Geometry: final body of the model. Coordinates: model frame, mm. A direction names the side the tool comes from. Coordinates: 2 decimals unless noted, no trailing zeros. Write each loop counter-clockwise with the first axis right and the second up, starting at its lowest first coordinate (ties: lowest second). Pieces come first, ordered by that corner, then holes. Notation, with made-up numbers: (75.5, 81.5) -> (124.5, 81.5) arc R20 ccw to (124.5, 88.5) -> close; hole circle Ø4 at (49.25, -35). An arc over 180 degrees is marked (long way). One line per item, written item: value.
```python
from build123d import *

# Parameters (mm, degrees)
EXTRUDE_1_DEPTH                = 15
SKETCH_2_R                     = 1.5
EXTRUDE_2_DEPTH                = 6
SKETCH_3_R                     = 1.5
SKETCH_3_R_2                   = 1.25
CUT_EXTRUDE_3_DEPTH            = 0.5
CHAMFER_1_SIZE                 = 0.2
M4_CLEARANCE_HOLE1_D           = 2.5
M4_CLEARANCE_HOLE1_DEPTH       = 6
M4_CLEARANCE_HOLE1_CSINK_D     = 3
M4_CLEARANCE_HOLE1_CSINK_ANGLE = 90
M4_CLEARANCE_HOLE1_TIP         = 0.751075774


with BuildPart() as part:
    # Эскиз1 → Вытянуть1 (new body)
    with BuildSketch(Plane.XY):
        Polygon((0, 2.886751346), (-2.5, 1.443375673), (-2.5, -1.443375673), (0, -2.886751346), (2.5, -1.443375673), (2.5, 1.443375673), align=None)
    extrude(amount=EXTRUDE_1_DEPTH)

    # Эскиз2 → Вытянуть2 (add)
    with BuildSketch(Plane.XY.offset(15)):
        Circle(SKETCH_2_R)
    extrude(amount=EXTRUDE_2_DEPTH)

    # Эскиз3 → Вырез-Вытянуть3 (cut)
    with BuildSketch(Plane.XY.offset(15)):
        Circle(SKETCH_3_R)
        Circle(SKETCH_3_R_2, mode=Mode.SUBTRACT)
    extrude(amount=CUT_EXTRUDE_3_DEPTH, mode=Mode.SUBTRACT)

    # Фаска1
    chamfer_1_edges = [part.edges().sort_by_distance(p)[0] for p in [
        (-1.5, 0, 21),
        (-1.5, 0, 15.5),
    ]]
    chamfer(chamfer_1_edges, length=CHAMFER_1_SIZE)

    # M4 Clearance Hole1
    with Locations(Plane(origin=(0, 0, 0), x_dir=(-1, 0, 0), z_dir=(0, 0, -1))):
        with Locations((0, 0)):
            CounterSinkHole(M4_CLEARANCE_HOLE1_D / 2, M4_CLEARANCE_HOLE1_CSINK_D / 2, depth=M4_CLEARANCE_HOLE1_DEPTH, counter_sink_angle=M4_CLEARANCE_HOLE1_CSINK_ANGLE)
            with Locations((0, 0, -(M4_CLEARANCE_HOLE1_DEPTH + M4_CLEARANCE_HOLE1_TIP / 2))):  # 118° drill point
                Cone(0, M4_CLEARANCE_HOLE1_D / 2, M4_CLEARANCE_HOLE1_TIP, mode=Mode.SUBTRACT)


solid = part.part
```
(1) Section A-A (z = 14.25). Return the cut outline in (x, y), then the cut area to 3 significant figures.
Responses:
outline: (-2.5, -1.44) -> (0, -2.89) -> (2.5, -1.44) -> (2.5, 1.44) -> (0, 2.89) -> (-2.5, 1.44) -> close
area: 21.7 mm2
(2) Section D-D (z = 18.25). Return the cut outline in (x, y).
Responses:
outline: circle Ø3 at (0, 0)
(3) Section C-C (y = -1.9). Return the cut outline in (x, z), then the cut area to 3 significant figures.
Responses:
outline: (-1.71, 0) -> (1.71, 0) -> (1.71, 15) -> (-1.71, 15) -> close
area: 51.3 mm2
(4) Pull-direction query (X, two-part tool) for faces 1 (the flat face through (-2.5, 0, 7)), 2 (the flat face through (-1, -1, 15)), 3 (the cylindrical face through (-0.27, -1.22, 3.17)); classes: released by +X, released by -X, zero draft, split by the parting line, or undercut.
Responses:
face 1: released by -X
face 2: zero draft
face 3: undercut
(5) Reachability of faces 4 (the cylindrical face through (-1.5, 0.07, 18.21)), 5 (the flat face through (2.5, 0, 7)), 6 (the cylindrical face through (-0.27, -1.22, 15.25)) from +Z, -Z, +X, -X, +Y, -Y: full face, straight path, thin tool, end or side. Return the list, or none.
Responses:
face 4: +Z
face 5: +Z, -Z, +X, +Y, -Y
face 6: none
(6) Section B-B (z = 6.25). Return the cut outline in (x, y).
Responses:
outline: (-2.5, -1.44) -> (0, -2.89) -> (2.5, -1.44) -> (2.5, 1.44) -> (0, 2.89) -> (-2.5, 1.44) -> close; hole circle Ø1.67 at (0, 0)
(7) Line query: line 1 (X direction, y = 0, z = 3.45); line 2 (Z direction, x = -2.1, y = -0.45); line 3 (X direction, y = 0.95, z = 5.5). Output: solid intervals per line, ascending. Write a range as [from, to].
Responses:
line 1: x = [-2.5, -1.25], [1.25, 2.5]
line 2: z = [0, 15]
line 3: x = [-2.5, -0.81], [0.81, 2.5]
(8) First-contact query: pin 1 (1 mm diameter, centred on x = -2, z = 10, fed in from +Y); pin 2 (2 mm diameter, centred on x = -2, z = 9, fed in from +Y). Flat tips, straight axial feed; report the tip coordinate or a pass-through.
Responses:
pin 1: stops at y = 2.02
pin 2: stops at y = 2.31
